Source: CAD feature listing. Evaluate the final solid. Frame: model axes, mm. Face numbers are marked on the shaded views. A direction names the side the tool comes from. Round coordinates to 2 decimals unless told otherwise and drop trailing zeros. Write each loop counter-clockwise with the first axis right and the second up, starting at its lowest first coordinate (ties: lowest second). Pieces come first, ordered by that corner, then holes.
from build123d import *

# Parameters (mm, degrees)
BOSS_EXTRUDE1_DEPTH     = 7.7
SKETCH2_W               = 7
SKETCH2_H               = 3.1
CUT_EXTRUDE1_DEPTH      = 79.027559234
FILLET1_R               = 10
BOSS_EXTRUDE2_DEPTH     = 6
BOSS_EXTRUDE4_REACH     = 122.547
CUT_EXTRUDE2_DEPTH      = 121.437504541
CUT_EXTRUDE2_DEPTH_BACK = 121.437504541
CUT_EXTRUDE3_DEPTH      = 10
FILLET3_R               = 1
FILLET5_R               = 3
CUT_EXTRUDE4_REACH      = 123.217
SKETCH8_W               = 17
SKETCH8_H               = 5
SKETCH8_W_2             = 19
SKETCH8_H_2             = 7
FILLET6_R               = 2
FILLET7_R               = 2
BOSS_EXTRUDE5_DEPTH     = 2.5
FILLET8_R               = 5
SKETCH11_R              = 1
CUT_EXTRUDE5_DEPTH      = 0.7
SKETCH13_W              = 22.342383579
SKETCH13_H              = 4
CUT_EXTRUDE6_DEPTH      = 2
SKETCH14_W              = 66.9
SKETCH14_H              = 84.5
CUT_EXTRUDE8_DEPTH      = 5


with BuildPart() as part:
    # Sketch1 → Boss-Extrude1 (new body)
    with BuildSketch(Plane(origin=(0, 0, 0), x_dir=(1, 0, 0), z_dir=(0, 1, 0))):
        Polygon((0, 0), (-16.35, 0), (-16.35, -9.85), (-2.6, -9.85), (-2.6, -33), (-20.1, -33), (-20.1, -75), (0, -75), align=None)
    extrude(amount=BOSS_EXTRUDE1_DEPTH)

    # Sketch2 → Cut-Extrude1 (cut, through all)
    with BuildSketch(Plane.XY.offset(75)):
        with Locations((-16.6, 3.55)):
            Rectangle(SKETCH2_W, SKETCH2_H)
    extrude(amount=-CUT_EXTRUDE1_DEPTH, mode=Mode.SUBTRACT)

    # Fillet1
    fillet1_edges = [part.edges().sort_by_distance(p)[0] for p in [
        (-2.6, 3.85, 33),
    ]]
    fillet(fillet1_edges, radius=FILLET1_R)

    # Sketch3 → Boss-Extrude2 (add)
    with BuildSketch(Plane(origin=(0, 7.7, 0), x_dir=(1, 0, 0), z_dir=(0, 1, 0))):
        Polygon((0, 4.5), (-33.45, 4.5), (-33.45, -75), (-10, -115), (0, -115), align=None)
    extrude(amount=BOSS_EXTRUDE2_DEPTH)

    # Boss-Extrude4: up to this face of the body (flat: up to its plane)
    boss_extrude4_end = Plane(part.part.faces().sort_by_distance((0, 7.644090382, 47.331402086))[0])
    # Sketch5 → Boss-Extrude4 (add, up to the picked face)
    with BuildSketch(Plane.ZY.offset(33.45), mode=Mode.PRIVATE) as boss_extrude4_sk1:
        Polygon((75, 7.7), (75, -5), (90, -5), (115, 7.7), align=None)
    boss_extrude4_tool1 = split(extrude(boss_extrude4_sk1.sketch, amount=-BOSS_EXTRUDE4_REACH, mode=Mode.PRIVATE), bisect_by=boss_extrude4_end, keep=Keep.BOTH, mode=Mode.PRIVATE)
    add(boss_extrude4_tool1.solids().sort_by(Axis((-33.45, 2.312121, 89.69697), (1, 0, 0)))[0])

    # Sketch6 → Cut-Extrude2 (cut, two sides: drawn at the far end of the back side and taken through both)
    with BuildSketch(Plane(origin=(0, 7.7, 0), x_dir=(1, 0, 0), z_dir=(0, 1, 0)).offset(-CUT_EXTRUDE2_DEPTH_BACK)):
        Polygon((-33.45, -75), (-10, -115), (-33.45, -115), align=None)
    extrude(amount=CUT_EXTRUDE2_DEPTH + CUT_EXTRUDE2_DEPTH_BACK, mode=Mode.SUBTRACT)

    # Sketch7 → Cut-Extrude3 (cut)
    with BuildSketch(Plane(origin=(0, 0, 0), x_dir=(0, 0, -1), z_dir=(1, 0, 0))):
        Polygon((-75, 0), (-82, 0), (-80, -5), (-75, -5), align=None)
    extrude(amount=-CUT_EXTRUDE3_DEPTH, mode=Mode.SUBTRACT)

    # Fillet3
    fillet3_edges = [part.edges().sort_by_distance(p)[0] for p in [
        (-10, -5, 77.5),
        (-5, -5, 80),
    ]]
    fillet(fillet3_edges, radius=FILLET3_R)

    # Mirror1: part across plane


with BuildPart() as part_1:
    add(part.part)
    add(part.part.mirror(Plane(origin=(0, 7.7, 75), x_dir=(0, 0, 1), z_dir=(-1, 0, 0))))

    # Fillet5
    fillet5_edges = [part_1.edges().sort_by_distance(p)[0] for p in [
        (-29.053125, -5, 82.5),
        (29.053125, -5, 82.5),
    ]]
    fillet(fillet5_edges, radius=FILLET5_R)

    # Cut-Extrude4: up to this face of the body (flat: up to its plane)
    cut_extrude4_end = Plane(part_1.part.faces().sort_by_distance((0, 0, 46.525100135))[0])
    # Sketch8 → Cut-Extrude4 (cut, up to the picked face)
    with BuildSketch(Plane(origin=(0, 13.7, 0), x_dir=(1, 0, 0), z_dir=(0, 1, 0)), mode=Mode.PRIVATE) as cut_extrude4_sk1:
        with Locations((24.95, 2)):
            Rectangle(SKETCH8_W, SKETCH8_H)
    cut_extrude4_tool1 = split(extrude(cut_extrude4_sk1.sketch, amount=-CUT_EXTRUDE4_REACH, mode=Mode.PRIVATE), bisect_by=cut_extrude4_end, keep=Keep.BOTH, mode=Mode.PRIVATE)
    # Sketch8 → Cut-Extrude4 (cut, up to the picked face)
    with BuildSketch(Plane(origin=(0, 13.7, 0), x_dir=(1, 0, 0), z_dir=(0, 1, 0)), mode=Mode.PRIVATE) as cut_extrude4_sk2:
        with Locations((-24.95, 2)):
            Rectangle(SKETCH8_W_2, SKETCH8_H_2)
    cut_extrude4_tool2 = split(extrude(cut_extrude4_sk2.sketch, amount=-CUT_EXTRUDE4_REACH, mode=Mode.PRIVATE), bisect_by=cut_extrude4_end, keep=Keep.BOTH, mode=Mode.PRIVATE)
    add(cut_extrude4_tool1.solids().sort_by(Axis((24.95, 13.7, -2), (0, -1, 0)))[0], mode=Mode.SUBTRACT)
    add(cut_extrude4_tool2.solids().sort_by(Axis((-24.95, 13.7, -2), (0, -1, 0)))[0], mode=Mode.SUBTRACT)

    # Fillet6
    fillet6_edges = [part_1.edges().sort_by_distance(p)[0] for p in [
        (-15.45, 10.7, -4.5),
        (-33.45, 10.7, 1.5),
    ]]
    fillet(fillet6_edges, radius=FILLET6_R)

    # Fillet7
    fillet7_edges = [part_1.edges().sort_by_distance(p)[0] for p in [
        (33.45, 10.7, 0.5),
        (16.45, 10.7, -4.5),
    ]]
    fillet(fillet7_edges, radius=FILLET7_R)

    # Sketch12 → Boss-Extrude5 (add, symmetric)
    with BuildSketch(Plane.ZY.offset(-0.2)):
        Polygon((93.346456693, -3.3), (108.972772013, 4.638168182), (104.121669234, -3.3), align=None)
    extrude(amount=BOSS_EXTRUDE5_DEPTH, both=True)

    # Fillet8
    fillet8_edges = [part_1.edges().sort_by_distance(p)[0] for p in [
        (0.2, -3.3, 104.121669234),
    ]]
    fillet(fillet8_edges, radius=FILLET8_R)

    # Sketch11 → Cut-Extrude5 (cut)
    with BuildSketch(Plane.ZY.offset(-0.2)):
        with Locations((82.490949754, -1.3)):
            Circle(SKETCH11_R)
        with Locations((103, -1.3)):
            Circle(SKETCH11_R)
        Polygon((82.490949754, -1.3), (103, -1.3), (114, 16.7), (93.490949754, 16.7), align=None)
        with BuildLine():
            Line((83.490949754, -1.3), (82.490949754, -1.3))
            Line((82.490949754, -1.3), (83.012399764, -0.446718166))
            ThreePointArc((83.012399764, -0.446718166), (81.618754246, -1.789157434), (83.490949754, -1.3))
        make_face()
        with BuildLine():
            Line((83.012399764, -0.446718166), (82.490949754, -1.3))
            Line((82.490949754, -1.3), (83.490949754, -1.3))
            ThreePointArc((83.490949754, -1.3), (83.363145263, -0.810842566), (83.012399764, -0.446718166))
        make_face()
        with BuildLine():
            ThreePointArc((103.521450009, -0.446718166), (102.510842566, -0.427804492), (102, -1.3))
            Line((102, -1.3), (103, -1.3))
            Line((103, -1.3), (103.521450009, -0.446718166))
        make_face()
        with BuildLine():
            Line((103, -1.3), (102, -1.3))
            ThreePointArc((102, -1.3), (103, -2.3), (104, -1.3))
            ThreePointArc((104, -1.3), (103.872195508, -0.810842566), (103.521450009, -0.446718166))
            Line((103.521450009, -0.446718166), (103, -1.3))
        make_face()
    extrude(amount=-CUT_EXTRUDE5_DEPTH, mode=Mode.SUBTRACT)

    # Sketch13 → Cut-Extrude6 (cut)
    with BuildSketch(Plane.ZY.offset(-0.2)):
        with Locations((102.828808211, 11.7)):
            Rectangle(SKETCH13_W, SKETCH13_H)
    extrude(amount=CUT_EXTRUDE6_DEPTH, mode=Mode.SUBTRACT)

    # Sketch14 → Cut-Extrude8 (cut)
    with BuildSketch(Plane(origin=(0, 13.7, 0), x_dir=(1, 0, 0), z_dir=(0, 1, 0))):
        with Locations((0, -37.75)):
            Rectangle(SKETCH14_W, SKETCH14_H)
    extrude(amount=-CUT_EXTRUDE8_DEPTH, mode=Mode.SUBTRACT)


solid = part_1.part
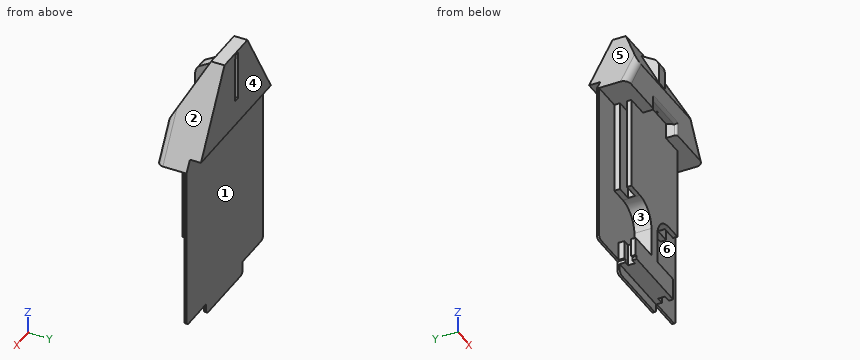
1) Contact query for flat-ended pins moving along their axis: P1, Ø1.5, axis at y = 4, z = 56, coming from the +X side; P2, Ø8, axis at y = 7, z = 100, coming from the -X side; P3, Ø1.5, axis at x = -17.5, z = 72.5, coming from the -Y side. Output: stop coordinate, or through.
Taken from the geometry:
P1: stops at x = 13.1
P2: stops at x = -21.14
P3: stops at y = 0
2) Section query A-A on z = 7.5. Return the cut outline in (x, y), then the cut area to 3 significant figures.
Taken from the geometry:
outline: (-33.45, 7.7) - (-16.35, 7.7) - (-16.35, 5.1) - (-13.1, 5.1) - (-13.1, 2) - (-16.35, 2) - (-16.35, 0) - (16.35, 0) - (16.35, 2) - (13.1, 2) - (13.1, 5.1) - (16.35, 5.1) - (16.35, 7.7) - (33.45, 7.7) - (33.45, 8.7) - (-33.45, 8.7) - close
area: 299 mm2
3) Reachability of the marked faces 1 and 2 from +Z, -Z, +X, -X, +Y, -Y: full face, straight path, thin tool, end or side. Return the list, or none.
Taken from the geometry:
face 1: -Z, +X, -X, +Y
face 2: +Z, +X, +Y, -Y
4) Material intervals for line 1 (Y direction, x = -26, z = 39.5); line 2 (Y direction, x = 10.5, z = 55); line 3 (X direction, y = 3, z = 60.5), sorted ascending.
Taken from the geometry:
line 1: y = 7.7 to 8.7
line 2: y = 0 to 8.7
line 3: x = -13.1 to 13.1
5) Section query B-B on z = 55. Return the cut outline in (x, y), then the cut area to 3 significant figures.
Taken from the geometry:
outline: (-33.45, 7.7) - (-20.1, 7.7) - (-20.1, 5.1) - (-13.1, 5.1) - (-13.1, 2) - (-20.1, 2) - (-20.1, 0) - (20.1, 0) - (20.1, 2) - (13.1, 2) - (13.1, 5.1) - (20.1, 5.1) - (20.1, 7.7) - (33.45, 7.7) - (33.45, 8.7) - (-33.45, 8.7) - close
area: 333 mm2
6) Pull-direction query (Z, two-part tool) for the marked faces 3, 4, 5 and 6; classes: released by +Z, released by -Z, zero draft, split by the parting line, or undercut.
Taken from the geometry:
face 3: undercut
face 4: zero draft
face 5: released by +Z
face 6: undercut
